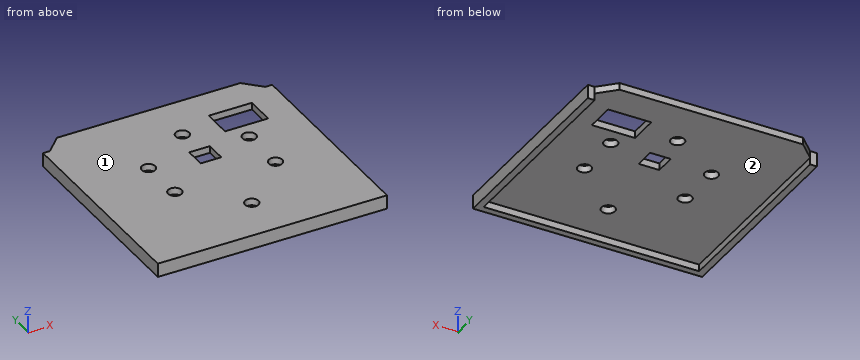
```python
from build123d import *

# Parameters (mm, degrees)
CROQUIS1_R              = 2.950001172
CROQUIS1_W              = 9
CROQUIS1_H              = 9
CROQUIS1_W_2            = 18.849999644
CROQUIS1_H_2            = 12.749999762
SALIENTE_EXTRUIR1_DEPTH = 3
SALIENTE_EXTRUIR6_DEPTH = 3


with BuildPart() as part:
    # Croquis1 → Saliente-Extruir1 (new body)
    with BuildSketch(Plane.XY.offset(-0.156260387)):
        Polygon((51.261125499, 62.988673094), (44.261125499, 69.988673094), (-35.738874501, 69.988673094), (-42.738874501, 62.988673094), (-45.738874501, 62.988673094), (-45.738874501, -27.011326906), (54.261125499, -27.011326906), (54.261125499, 62.988673094), align=None)
        with Locations((7.161124531, 48.770443145)):
            Circle(CROQUIS1_R, mode=Mode.SUBTRACT)
        with Locations((28.761125092, 35.170443896)):
            Circle(CROQUIS1_R, mode=Mode.SUBTRACT)
        with Locations((28.761125092, 14.5704435)):
            Circle(CROQUIS1_R, mode=Mode.SUBTRACT)
        with Locations((6.661127243, -6.529559074)):
            Circle(CROQUIS1_R, mode=Mode.SUBTRACT)
        with Locations((-15.198872503, 14.470443669)):
            Circle(CROQUIS1_R, mode=Mode.SUBTRACT)
        with Locations((-15.738875683, 34.170445595)):
            Circle(CROQUIS1_R, mode=Mode.SUBTRACT)
        with Locations((7.748576734, 31.892113927)):
            Rectangle(CROQUIS1_W, CROQUIS1_H, mode=Mode.SUBTRACT)
        with Locations((31.861125879, 49.188674036)):
            Rectangle(CROQUIS1_W_2, CROQUIS1_H_2, mode=Mode.SUBTRACT)
    extrude(amount=SALIENTE_EXTRUIR1_DEPTH)

    # Croquis9 → Saliente-Extruir6 (add)
    with BuildSketch(Plane(origin=(0, 0, -0.156260387), x_dir=(-1, 0, 0), z_dir=(0, 0, -1))):
        Polygon((-54.261125499, 62.988673094), (-51.261125499, 62.988673094), (-51.261125499, -24.011326906), (42.738874501, -24.011326906), (42.738874501, 62.988673094), (45.738874501, 62.988673094), (45.738874501, -27.011326906), (-54.261125499, -27.011326906), align=None)
    extrude(amount=SALIENTE_EXTRUIR6_DEPTH)


solid = part.part
```
Geometry: final body of the model. Coordinates: model frame, mm. Face numbers are marked on the shaded views. Coordinates: 2 decimals unless noted, no trailing zeros. Order: outer loops, then holes, each group sorted by start corner. A loop starts at its lowest first (then second) coordinate and runs counter-clockwise, first axis right, second up. Notation, with made-up numbers: (84, -13) - (117, -13) arc R20 cw to (117, 8) - close; hole circle Ø1 at (84, 71.5). An arc over 180 degrees is marked (long way). Write each question's results on one line, items separated by ' | '.
(1) Section query A-A, the plane y = -19. Return the cut outline in (x, z).
Values found:
outline: (-45.74, -3.16) - (-42.74, -3.16) - (-42.74, -0.16) - (51.26, -0.16) - (51.26, -3.16) - (54.26, -3.16) - (54.26, 2.84) - (-45.74, 2.84) - close
(2) Section query B-B, the plane x = 35. Return the cut outline in (y, z).
Values found:
outline: (-27.01, -3.16) - (-24.01, -3.16) - (-24.01, -0.16) - (42.81, -0.16) - (42.81, 2.84) - (-27.01, 2.84) - close; (55.56, -0.16) - (69.99, -0.16) - (69.99, 2.84) - (55.56, 2.84) - close
(3) Section query C-C, the plane z = -2.05. Return the cut outline in (x, y), plus the area to 3 significant figures.
Values found:
outline: (-45.74, -27.01) - (54.26, -27.01) - (54.26, 62.99) - (51.26, 62.99) - (51.26, -24.01) - (-42.74, -24.01) - (-42.74, 62.99) - (-45.74, 62.99) - close | area: 822 mm²
(4) Mould query, pull axis X, two halves, no side actions, for the marked faces 1 and 2. Classes: +X half, -X half, draft (parallel to the pull), parting line (faces both ways), or undercut.
Values found:
face 1: draft | face 2: undercut
(5) First-contact query: pin 1 Ø7.5 at (x, y) = (28.76, 14.57) entering from +Z; pin 2 Ø2.5 at (x, z) = (52.5, -0.5) entering from +Y; pin 3 Ø2 at (x, y) = (-26, 51) entering from -Z; pin 4 Ø0.9 at (x, z) = (-12.5, -1.5) entering from +Y. Flat tips, straight axial feed; report the tip coordinate or a pass-through.
Values found:
pin 1: stops at z = 2.84 | pin 2: stops at y = 62.99 | pin 3: stops at z = -0.16 | pin 4: stops at y = -24.01
(6) Section query D-D, the plane y = 47. Return the cut outline in (x, z).
Values found:
outline: (-45.74, -3.16) - (-42.74, -3.16) - (-42.74, -0.16) - (4.8, -0.16) - (4.8, 2.84) - (-45.74, 2.84) - close; (9.52, -0.16) - (22.44, -0.16) - (22.44, 2.84) - (9.52, 2.84) - close; (41.29, -0.16) - (51.26, -0.16) - (51.26, -3.16) - (54.26, -3.16) - (54.26, 2.84) - (41.29, 2.84) - close
(7) Line query: line 1 (X direction, y = 48.5, z = 0.35); line 2 (X direction, y = 61, z = -2.55); line 3 (Y direction, x = 3.5, z = 0). Output: solid intervals per line, ascending. Write a range as [from, to].
Values found:
line 1: x = [-45.74, 4.22], [10.1, 22.44], [41.29, 54.26] | line 2: x = [-45.74, -42.74], [51.26, 54.26] | line 3: y = [-27.01, 27.39], [36.39, 69.99]
